```python
from build123d import *

# Parameters (mm, degrees)
F1_DEPTH = 20
F4_R     = 9.99999
F6_D     = 3
F2_W     = 4
F2_H     = 10
F7_DEPTH = 25
F8_D     = 3


# Not quite as in the source:
# - a fillet or chamfer is up to 0.001 mm smaller than in the source, because OpenCascade refuses the exact size
# - a feature names something its author has since deleted; it is built from what else it names


with BuildPart() as f1:
    # F0 (on Top) → F1 (new body)
    with BuildSketch(Plane.XY):
        with BuildLine():
            Line((0, 2), (0, 0))
            Line((0, 0), (57, 0))
            ThreePointArc((57, 0), (62.6568542495, -2.3431457505), (65, -8))
            Line((65, -8), (65, -95))
            Line((65, -95), (67, -95))
            Line((67, -95), (67, -8))
            ThreePointArc((67, -8), (64.0710678119, -0.9289321881), (57, 2))
            Line((57, 2), (0, 2))
        make_face()
    extrude(amount=F1_DEPTH)

    # F4 (radius 10 in the source; OpenCascade refuses exactly that, so slightly less here)
    f4_edges = [f1.edges().sort_by_distance(p)[0] for p in [
        (0, 1, 20),
        (0, 1, 0),
        (66, -95, 20),
        (66, -95, 0),
    ]]
    fillet(f4_edges, radius=F4_R)

    # F6 (through all)
    with Locations(Plane(origin=(65, 0, 0), x_dir=(0, -1, 0), z_dir=(-1, 0, 0))):
        with Locations((80.7573593129, 14.2426406871), (80.7573593129, 5.7573593129), (89.2426406871, 5.7573593129), (89.2426406871, 14.2426406871)):
            Hole(F6_D / 2)

    # F2 (on face) → F7 (cut)
    with BuildSketch(Plane.XZ):
        with Locations((46, 10)):
            Rectangle(F2_W, F2_H)
    extrude(amount=-F7_DEPTH, mode=Mode.SUBTRACT)

    # F8 (through all)
    with Locations(Plane.XZ):
        with Locations((8.2824855787, 3.4264645687), (21.7175144213, 16.8614934112), (20.6568542495, 4.4871247404), (9.3431457505, 15.8008332394)):
            Hole(F8_D / 2)


solid = f1.part
```
Geometry: final body of the model. Coordinates: model frame, mm. A direction names the side the tool comes from. Round coordinates to 2 decimals unless told otherwise and drop trailing zeros. Write each loop counter-clockwise with the first axis right and the second up, starting at its lowest first coordinate (ties: lowest second). Pieces come first, ordered by that corner, then holes.
Item 1: Mould query, pull axis X, two halves, no side actions, for faces 4 (the face through (48, 1, 10)), 5 (the face through (66.01, -79.37, 13.67)), 6 (the face through (67, -52, 10)). Classes: +X half, -X half, draft (parallel to the pull), parting line (faces both ways), or undercut.
Item 2: Section query A-A (x = 46). Return loops of the section in (y, z).
Item 3: Section query B-B (x = 33). Return loops of the section in (y, z), plus the area to 3 significant figures.
Item 4: Section query C-C (y = -10.5). Return loops of the section in (x, z), plus the area to 3 significant figures.
Item 5: Set-up query: faces 1 (the face through (44, 1, 10)), 2 (the face through (28, 0, 10)), 3 (the face through (2.85, 0.99, 3.01)). Return all of +Z, -Z, +X, -X, +Y, -Y with unobstructed straight access to the full face (end or side cutting, diameter ignored); none if empty.
Item 6: Pin query (flat end, axial travel): P1, Ø1, axis at y = -84.5, z = 16, coming from the -X side; P2, Ø2.5, axis at y = -80.76, z = 14.24, coming from the -X side; P3, Ø4, axis at x = 56.5, z = 15.5, coming from the -Y side; P4, Ø2, axis at y = 1, z = 8, coming from the -X side. Return the tip coordinate at first contact, or that it passes through.
Item 7: Material intervals for L1, parallel to X at y = -13.5, z = 9; L2, parallel to Y at x = 16.5, z = 7.25; L3, parallel to Y at x = 63, z = 7, sorted ascending.
Completed:
1. face 4: undercut
1. face 5: draft
1. face 6: +X half
2. outline: (0, 0) - (2, 0) - (2, 5) - (0, 5) - close; (0, 15) - (2, 15) - (2, 20) - (0, 20) - close
3. outline: (0, 0) - (2, 0) - (2, 20) - (0, 20) - close
3. area: 40.0 mm2
4. outline: (65, 0) - (67, 0) - (67, 20) - (65, 20) - close
4. area: 40.0 mm2
5. face 1: +Y, -Y
5. face 2: +Z, -Z, -X, -Y
5. face 3: -Z, -X, +Y, -Y
6. P1: stops at x = 65
6. P2: passes through
6. P3: stops at y = -0.14
6. P4: stops at x = 0.05
7. L1: x = 65 to 67
7. L2: y = 0 to 2
7. L3: y = -2.71 to 0
